```python
from build123d import *

# Parameters (mm, degrees)
SKETCH_1_W      = 30
SKETCH_1_H      = 10
EXTRUDE_1_DEPTH = 2


with BuildPart() as part:
    # 草图1 → 凸台-拉伸1 (new body)
    # profile 1 of 2: a face of its own
    with BuildSketch(Plane(origin=(0, 0, 0), x_dir=(1, 0, 0), z_dir=(0, 1, 0))):
        Rectangle(SKETCH_1_W, SKETCH_1_H)
        with BuildLine():
            Line((10, -2.5), (-10, -2.5))
            ThreePointArc((-10, -2.5), (-12.5, 0), (-10, 2.5))
            Line((-10, 2.5), (10, 2.5))
            ThreePointArc((10, 2.5), (11.767766953, 1.767766953), (12.5, 0))
            ThreePointArc((12.5, 0), (11.767766953, -1.767766953), (10, -2.5))
        make_face(mode=Mode.SUBTRACT)
    # profile 2 of 2: a face of its own
    with BuildSketch(Plane(origin=(0, 0, 0), x_dir=(1, 0, 0), z_dir=(0, 1, 0))):
        with BuildLine():
            ThreePointArc((-7.5, 0), (-8.232233047, -1.767766953), (-10, -2.5))
            Line((-10, -2.5), (10, -2.5))
            ThreePointArc((10, -2.5), (7.5, 0), (10, 2.5))
            Line((10, 2.5), (-10, 2.5))
            ThreePointArc((-10, 2.5), (-8.232233047, 1.767766953), (-7.5, 0))
        make_face()
    extrude(amount=EXTRUDE_1_DEPTH)


solid = part.part
```
Verification items for the finished model (mm, model axes). Coordinates: 2 decimals unless noted, no trailing zeros. Loops run counter-clockwise (first coordinate to the right, second up) from the corner with the lowest first, then second, coordinate; pieces in that order, holes last. Notation, with made-up numbers: (62.25, 36) -> (80.25, 36) arc R22 ccw to (80.25, 68) -> close; hole circle Ø1 at (-27, -37). An arc over 180 degrees is marked (long way). Answer in a Markdown table with one row per item. Add a question column.
1. Section check D-D, the plane x = -9.25. Enter the section's corners in (y, z), then the cut area to 3 significant figures.
2. Section check C-C, the plane y = 0.45. Enter the section's corners in (x, z), then the cut area to 3 significant figures.
3. Section check B-B, the plane z = -2. Enter the section's corners in (x, y), then the cut area to 3 significant figures.
4. Depth check by flat-ended pin: P1, Ø1, axis at x = -6.5, z = -3.5, coming from the -Y side. Enter the tip coordinate at first touch or a pass-through.
5. Section check A-A, the plane x = 12. Enter the section's corners in (y, z).
6. Material ranges on probe 1 along X at (y, z) = (1.85, 1.75); probe 2 along X at (y, z) = (1.15, 0.5); probe 3 along Z at (x, y) = (-8.25, 0.4), recorded low to high. Write a range as [from, to].
Derived:
| question | item | result |
|---|---|---|
| 1 | outline | (0, -5) -> (2, -5) -> (2, -2.38) -> (0, -2.38) -> close; (0, 2.38) -> (2, 2.38) -> (2, 5) -> (0, 5) -> close |
| 1 | area | 10.5 mm² |
| 2 | outline | (-15, -5) -> (15, -5) -> (15, 5) -> (-15, 5) -> close; hole circle Ø5 at (-10, 0); hole circle Ø5 at (10, 0) |
| 2 | area | 261 mm² |
| 3 | outline | (-15, 0) -> (-11.5, 0) -> (-11.5, 2) -> (-15, 2) -> close; (-8.5, 0) -> (8.5, 0) -> (8.5, 2) -> (-8.5, 2) -> close; (11.5, 0) -> (15, 0) -> (15, 2) -> (11.5, 2) -> close |
| 3 | area | 48.0 mm² |
| 4 | P1 | stops at y = 0 |
| 5 | outline | (0, -5) -> (2, -5) -> (2, -1.5) -> (0, -1.5) -> close; (0, 1.5) -> (2, 1.5) -> (2, 5) -> (0, 5) -> close |
| 6 | probe 1 | x = [-15, -11.79], [-8.21, 8.21], [11.79, 15] |
| 6 | probe 2 | x = [-15, -12.45], [-7.55, 7.55], [12.45, 15] |
| 6 | probe 3 | z = [-5, -1.79], [1.79, 5] |
